CAD build for the part. Positions are in the model's coordinates, mm. A direction names the side the tool comes from. Give positions to 0.01 mm unless a question says otherwise; leave off trailing zeros. Order: outer loops, then holes, each group sorted by start corner. A loop starts at its lowest first (then second) coordinate and runs counter-clockwise, first axis right, second up.
Item 1: Band-saw the part on B-B on x = 64. Give the cut face in (y, z).
Item 2: Two-plate mould, pull along X, no slides. Class faces 1 (the cylindrical face through (-29.2, 35.07, 107.34)), 2 (the cylindrical face through (-29.2, -34.93, 107.34)), 3 (the flat face through (80, 1, 1)), 4 (the cylindrical face through (39.44, -0.88, -39.99)): released by +X, released by -X, zero draft, split by the parting line, or undercut.
Item 3: Band-saw the part on D-D on z = 29. Give the cut face in (x, y), plus the area to 3 significant figures.
Item 4: Flat gauge pins, fed straight in: P1, Ø6, axis at x = 81.5, y = -5.5, coming from the +Z side; P2, Ø5, axis at y = -8, z = 39, coming from the +X side; P3, Ø12, axis at y = 20, z = 32, coming from the -X side; P4, Ø8, axis at y = -18.5, z = 47, coming from the -X side. Where does each tip first touch, or does it go through?
Item 5: Wall check: L1, parallel to Y at x = 27.5, z = 59; L2, parallel to X at y = 37, z = -10; L3, parallel to Z at x = 10.5, y = 34.5. Give the ranges that are in metal, low to high.
Item 6: Band-saw the part on C-C on y = 33. Give the cut face in (x, z).
Item 7: Which spindle directions (+Z, -Z, +X, -X, +Y, -Y) get a long thin tool onto all of the face, cutting with end or side? Do faces 5 (the flat face through (39, -40, 59)), 6 (the flat face through (0, 1, 1)), 7 (the flat face through (41, 0, 40)). Say none if no direction does.
Item 8: Band-saw the part on A-A on z = 90. Give the cut face in (x, y), plus the area to 3 significant figures.
```python
from build123d import *

# Parameters (mm, degrees)
BOSS_EXTRUDE1_DEPTH = 80
BOSS_EXTRUDE2_DEPTH = 80
SKETCH3_W           = 80
SKETCH3_H           = 60
CUT_EXTRUDE1_DEPTH  = 133


with BuildPart() as part:
    # Sketch1 → Boss-Extrude1 (new body)
    with BuildSketch(Plane(origin=(0, 0, 0), x_dir=(0, 0, -1), z_dir=(1, 0, 0))):
        with BuildLine():
            Line((0, 40), (-80, 40))
            Line((-80, 40), (-80, -40))
            Line((-80, -40), (0, -40))
            ThreePointArc((0, -40), (40, 0), (0, 40))
        make_face()
    extrude(amount=BOSS_EXTRUDE1_DEPTH)

    # Sketch2 → Boss-Extrude2 (add)
    with BuildSketch(Plane(origin=(0, 40, 0), x_dir=(1, 0, 0), z_dir=(0, 1, 0))):
        with BuildLine():
            Line((0, -80), (40, -80))
            ThreePointArc((40, -80), (28.284271247, -51.715728753), (0, -40))
            Line((0, -40), (0, -80))
        make_face()
        with BuildLine():
            ThreePointArc((0, -40), (-28.284271247, -108.284271247), (40, -80))
            Line((40, -80), (0, -80))
            Line((0, -80), (0, -40))
        make_face()
        with BuildLine():
            Line((80, -80), (40, -80))
            ThreePointArc((40, -80), (80, -120), (120, -80))
            ThreePointArc((120, -80), (108.284271247, -51.715728753), (80, -40))
            Line((80, -40), (80, -80))
        make_face()
        with BuildLine():
            ThreePointArc((80, -40), (51.715728753, -51.715728753), (40, -80))
            Line((40, -80), (80, -80))
            Line((80, -80), (80, -40))
        make_face()
    extrude(amount=-BOSS_EXTRUDE2_DEPTH)

    # Sketch3 → Cut-Extrude1 (cut, symmetric)
    with BuildSketch(Plane(origin=(80, 0, 0), x_dir=(0, 0, -1), z_dir=(1, 0, 0))):
        with Locations((-80, 0)):
            Rectangle(SKETCH3_W, SKETCH3_H)
    extrude(amount=CUT_EXTRUDE1_DEPTH, both=True, mode=Mode.SUBTRACT)


solid = part.part
```
The answers:
1. outline: (-40, 0) arc R40 ccw to (40, 0) - (40, 116.66) - (30, 116.66) - (30, 40) - (-30, 40) - (-30, 116.66) - (-40, 116.66) - close
2. face 1: undercut
2. face 2: undercut
2. face 3: released by +X
2. face 4: zero draft
3. outline: (0, -40) - (80, -40) - (80, 40) - (0, 40) - close
3. area: 6,400 mm2
4. P1: stops at z = 40
4. P2: stops at x = 80
4. P3: stops at x = 0
4. P4: passes through
5. L1: y = -40 to -30, 30 to 40
5. L2: x = 0 to 80
5. L3: z = -20.24 to 118.6
6. outline: (0, -22.61) - (80, -22.61) - (80, 40) arc R40 ccw (long way) to (40, 80) arc R40 ccw (long way) to (0, 40) - close
7. face 5: +Z, -Z, +X, -X, -Y
7. face 6: -Z, -X, +Y, -Y
7. face 7: +Z, +X, -X
8. outline: (-38.73, -40) - (38.73, -40) - (38.73, -30) - (-38.73, -30) - close; (-38.73, 30) - (38.73, 30) - (38.73, 40) - (-38.73, 40) - close; (41.27, -40) - (118.73, -40) - (118.73, -30) - (41.27, -30) - close; (41.27, 30) - (118.73, 30) - (118.73, 40) - (41.27, 40) - close
8. area: 3,100 mm2
